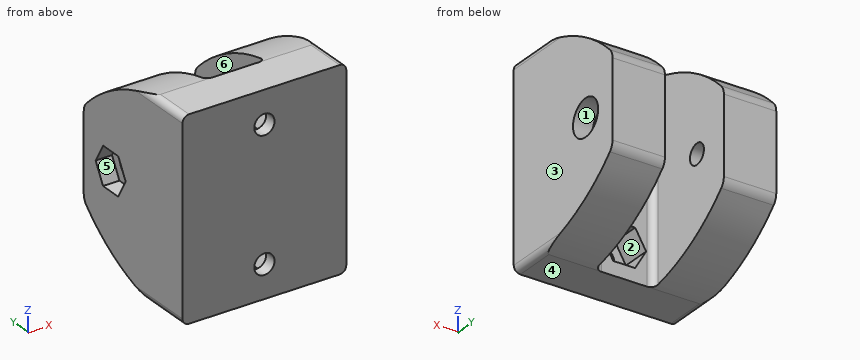
```python
from build123d import *

# Parameters (mm, degrees)
CROQUIS1_W              = 25
CROQUIS1_H              = 30
CROQUIS1_R              = 1.55
SALIENTE_EXTRUIR1_DEPTH = 22
CROQUIS2_W              = 9
CROQUIS2_H              = 15.632666969
CORTAR_EXTRUIR1_DEPTH   = 30
CROQUIS3_R              = 1.55
CORTAR_EXTRUIR2_DEPTH   = 25
CORTAR_EXTRUIR3_DEPTH   = 2.5
CROQUIS5_R              = 2.8
CORTAR_EXTRUIR4_DEPTH   = 3
CORTAR_EXTRUIR5_DEPTH   = 4.5
CORTAR_EXTRUIR6_DEPTH   = 25
REDONDEO1_R             = 2
REDONDEO2_R             = 1
REDONDEO3_R             = 1


with BuildPart() as part:
    # Croquis1 → Saliente-Extruir1 (new body)
    with BuildSketch(Plane(origin=(0, 0, 0), x_dir=(1, 0, 0), z_dir=(0, 1, 0))):
        with Locations((12.5, 15)):
            Rectangle(CROQUIS1_W, CROQUIS1_H)
        with Locations((12.5, 25)):
            Circle(CROQUIS1_R, mode=Mode.SUBTRACT)
        with Locations((12.5, 5)):
            Circle(CROQUIS1_R, mode=Mode.SUBTRACT)
    extrude(amount=SALIENTE_EXTRUIR1_DEPTH)

    # Croquis2 → Cortar-Extruir1 (cut)
    with BuildSketch(Plane(origin=(0, 0, -30), x_dir=(-1, 0, 0), z_dir=(0, 0, -1))):
        with Locations((-12.5, 14.183666516)):
            Rectangle(CROQUIS2_W, CROQUIS2_H)
    extrude(amount=-CORTAR_EXTRUIR1_DEPTH, mode=Mode.SUBTRACT)

    # Croquis3 → Cortar-Extruir2 (cut)
    with BuildSketch(Plane.ZY):
        with Locations((-15, 16)):
            Circle(CROQUIS3_R)
    extrude(amount=-CORTAR_EXTRUIR2_DEPTH, mode=Mode.SUBTRACT)

    # Croquis4 → Cortar-Extruir3 (cut)
    with BuildSketch(Plane.ZY):
        Polygon((-14.967896351, 19.348477667), (-17.8838149, 17.702041409), (-17.915918548, 14.353563741), (-15.032103649, 12.651522333), (-12.1161851, 14.297958591), (-12.084081452, 17.646436259), align=None)
    extrude(amount=-CORTAR_EXTRUIR3_DEPTH, mode=Mode.SUBTRACT)

    # Croquis5 → Cortar-Extruir4 (cut)
    with BuildSketch(Plane(origin=(25, 0, 0), x_dir=(0, 0, -1), z_dir=(1, 0, 0))):
        with Locations((15, 16)):
            Circle(CROQUIS5_R)
    extrude(amount=-CORTAR_EXTRUIR4_DEPTH, mode=Mode.SUBTRACT)

    # Croquis6 → Cortar-Extruir5 (cut)
    with BuildSketch(Plane(origin=(0, 6.367333031, 0), x_dir=(1, 0, 0), z_dir=(0, 1, 0))):
        Polygon((15.848631561, 25), (14.174315781, 27.9), (10.825684219, 27.9), (9.151368439, 25), (10.825684219, 22.1), (14.174315781, 22.1), align=None)
        Polygon((15.848631561, 5), (14.174315781, 7.9), (10.825684219, 7.9), (9.151368439, 5), (10.825684219, 2.1), (14.174315781, 2.1), align=None)
    extrude(amount=-CORTAR_EXTRUIR5_DEPTH, mode=Mode.SUBTRACT)

    # Croquis7 → Cortar-Extruir6 (cut)
    with BuildSketch(Plane.ZY):
        with BuildLine():
            Line((-21.708203932, 22), (-30, 22))
            Line((-30, 22), (-30, 6.37))
            ThreePointArc((-30, 6.37), (-27.145099003, 14.869880624), (-21.708203932, 22))
        make_face()
        with BuildLine():
            Line((0, 22), (-8.291796068, 22))
            ThreePointArc((-8.291796068, 22), (-2.854900997, 14.869880624), (0, 6.37))
            Line((0, 6.37), (0, 22))
        make_face()
    extrude(amount=-CORTAR_EXTRUIR6_DEPTH, mode=Mode.SUBTRACT)

    # Redondeo1
    redondeo1_edges = [part.edges().sort_by_distance(p)[0] for p in [
        (4, 22, -21.708203932),
        (21, 22, -21.708203932),
        (4, 22, -8.291796068),
        (21, 22, -8.291796068),
    ]]
    fillet(redondeo1_edges, radius=REDONDEO1_R)

    # Redondeo2
    redondeo2_edges = [part.edges().sort_by_distance(p)[0] for p in [
        (17, 6.367333031, -15),
        (8, 6.367333031, -15),
    ]]
    fillet(redondeo2_edges, radius=REDONDEO2_R)

    # Redondeo3
    redondeo3_edges = [part.edges().sort_by_distance(p)[0] for p in [
        (25, 3.185, -30),
        (0, 3.185, -30),
        (25, 3.185, 0),
        (0, 3.185, 0),
    ]]
    fillet(redondeo3_edges, radius=REDONDEO3_R)


solid = part.part
```
Could you check a few things on this model? Use its own coordinates, in mm. Face numbers are marked on the shaded views. A direction names the side the tool comes from. Give positions to 0.01 mm unless a question says otherwise; leave off trailing zeros. Write each loop counter-clockwise with the first axis right and the second up, starting at its lowest first coordinate (ties: lowest second). Pieces come first, ordered by that corner, then holes. Notation, with made-up numbers: (64, 51) - (91, 51) arc R22 ccw to (91, 77) - close; hole circle Ø4 at (-16.5, 3). An arc over 180 degrees is marked (long way). One line per item, written item: value. Start each with the question number.
Item 1: Imagine slicing it at D-D, the plane x = 21. List the corners of the cut face in (y, z) for me, and give its area (3 significant figures).
Item 2: Which directions (+Z, -Z, +X, -X, +Y, -Y) give clear straight access to the entire face, cutting with the end or side of a thin tool? Please do the marked faces 4, 5 and 6.
Item 3: If we mould it in two halves opening along X, with no side actions, what happens to the marked faces 1, 2 and 3? For each: +X half, -X half, draft (parallel to the pull), parting line (faces both ways), or undercut.
Item 4: Imagine slicing it at B-B, the plane y = 3. List the corners of the cut face in (x, z) for me.
Item 5: I'm going to push flat-ended pins straight in: pin 1 (4 mm diameter, centred on x = 16, z = -21.5, fed in from +Y); pin 2 (7.5 mm diameter, centred on x = 12, z = -19.5, fed in from +Y); pin 3 (4.5 mm diameter, centred on x = 12, z = -5, fed in from +Y); pin 4 (1.7 mm diameter, centred on y = 15, z = -16.5, fed in from +X). Where does each tip first touch, or does it pass through?
Item 6: Imagine slicing it at C-C, the plane y = 20.5. List the corners of the cut face in (x, z) for me, and give its area (3 significant figures).
Item 7: Please list where these lines run through material, in increasing order: line 1 (Z direction, x = 12.5, y = 0.6); line 2 (X direction, y = 14.25, z = -15.5); line 3 (X direction, y = 17, z = -8.5). Write a range as from..to.
Item 8: Imagine slicing it at A-A, the plane x = 12.5. List the corners of the cut face in (y, z) for me, and give its area (3 significant figures).
Geometry says:
1. outline: (0, -30) - (6.37, -30) arc R27.51 ccw to (21.41, -22.31) arc R2 ccw to (22, -20.9) - (22, -9.1) arc R2 ccw to (21.41, -7.69) arc R27.51 ccw to (6.37, 0) - (0, 0) - close; hole circle Ø3.1 at (16, -15)
1. area: 557 mm^2
2. face 4: -Z, +X, -X, +Y, -Y
2. face 5: -X
2. face 6: +Z, -Z, +Y
3. face 1: draft
3. face 2: undercut
3. face 3: +X half
4. outline: (0, -29) arc R1 ccw to (1, -30) - (24, -30) arc R1 ccw to (25, -29) - (25, -1) arc R1 ccw to (24, 0) - (1, 0) arc R1 ccw to (0, -1) - close; hole (9.15, -25) - (10.83, -27.9) - (14.17, -27.9) - (15.85, -25) - (14.17, -22.1) - (10.83, -22.1) - close; hole (9.15, -5) - (10.83, -7.9) - (14.17, -7.9) - (15.85, -5) - (14.17, -2.1) - (10.83, -2.1) - close
5. pin 1: y = 22
5. pin 2: y = 6.71
5. pin 3: y = 1.87
5. pin 4: x = 22
6. outline: (0, -23.18) - (8, -23.18) - (8, -6.82) - (0, -6.82) - close; (17, -23.18) - (25, -23.18) - (25, -6.82) - (17, -6.82) - close
6. area: 262 mm^2
7. line 1: -30..-26.55, -23.45..-6.55, -3.45..0
7. line 2: 2.5..8, 17..22
7. line 3: 0..8, 17..25
8. outline: (0, -30) - (6.37, -30) - (6.37, -27.9) - (1.87, -27.9) - (1.87, -26.55) - (0, -26.55) - close; (0, -23.45) - (1.87, -23.45) - (1.87, -22.1) - (6.37, -22.1) - (6.37, -7.9) - (1.87, -7.9) - (1.87, -6.55) - (0, -6.55) - close; (0, -3.45) - (1.87, -3.45) - (1.87, -2.1) - (6.37, -2.1) - (6.37, 0) - (0, 0) - close
8. area: 127 mm^2
